The figure shows three views and two pictorial views of one solid part (mm, origin at its lowest corner). Answer the questions. A direction names the side the tool comes from. Give positions to 0.01 mm unless a question says otherwise; leave off trailing zeros. Order: outer loops, then holes, each group sorted by start corner. A loop starts at its lowest first (then second) coordinate and runs counter-clockwise, first axis right, second up. Notation, with made-up numbers: M 53,-29.75 L 105,-29.75 A16 ccw 105,-2.75 Z; hole C -39,-0.75 d9. An arc over 180 degrees is marked long. Write item = value, one per line. Start each with the question number.
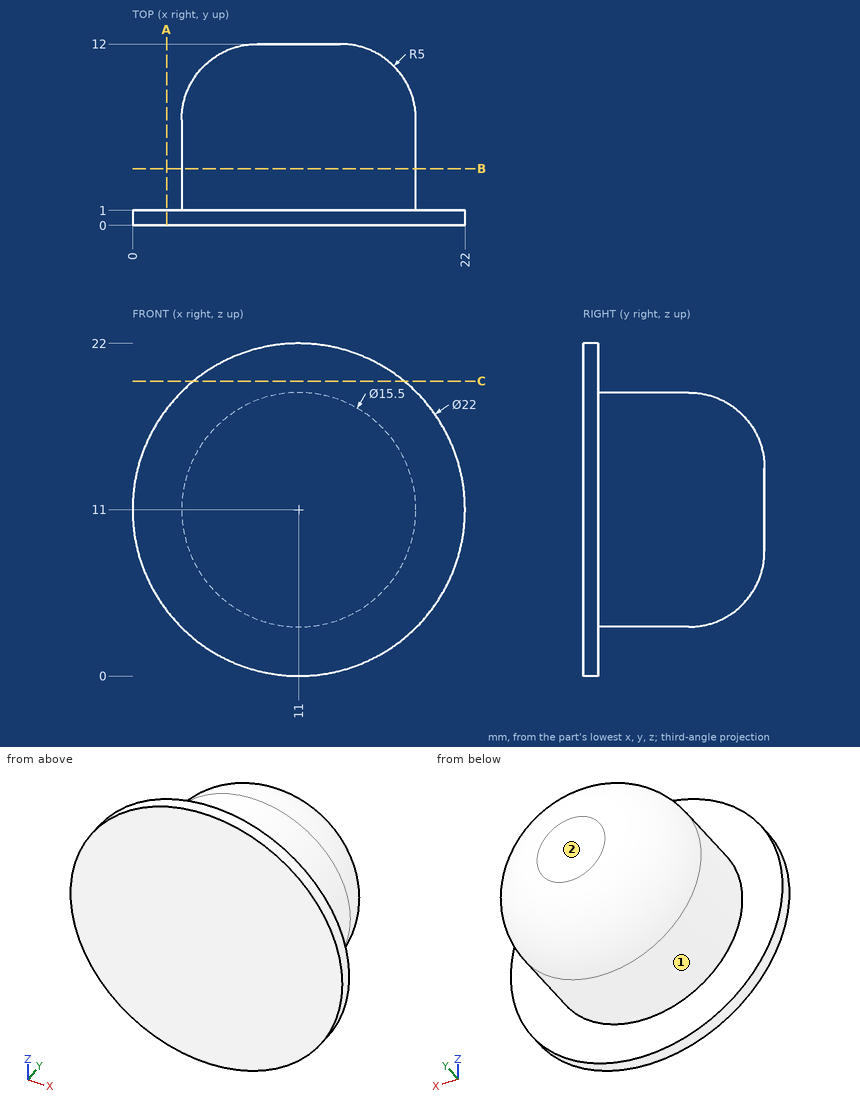
1) Find section C-C on z = 19.5. Determine the outline of the cut face in (x, y).
2) Each of these flat-tipped pins is pushed along its axis until it touches: P1, Ø3, axis at x = 11, y = 8, coming from the -Z side; P2, Ø3, axis at y = 5.5, z = 5.5, coming from the +X side; P3, Ø5, axis at x = 11.5, y = 11, coming from the +Z side. Where does it stop, or does it pass through?
3) For the marked faces 1 and 2, determine the directions among +Z, -Z, +X, -X, +Y, -Y from which every point of the face is accessible in a straight line to the end or side of a thin tool.
4) Find section B-B on y = 3.75. Determine the outline of the cut face in (x, z), plus the area to 3 significant figures.
5) Find the intervals of material crossed by probe 1 along Y at (x, z) = (4, 17.75); probe 2 along X at (y, z) = (9.75, 7.5); probe 3 along Y at (x, z) = (13.5, 4.5), in increasing order. Write a range as [from, to].
6) Find section A-A on x = 2.25. Determine the outline of the cut face in (y, z).
Numbers:
q1.outline = M 4.02,0 L 17.98,0 L 17.98,1 L 4.02,1 Z
q2.P1 = 3.25
q2.P2 = 17.64
q2.P3 = 18.51
q3.face_1 = +Y
q3.face_2 = +Z, -Z, +X, -X, +Y
q4.outline = C 11,11 d15.5
q4.area = 189 mm2
q5.probe_1 = [0, 1]
q5.probe_2 = [5.02, 16.98]
q5.probe_3 = [0, 9.69]
q6.outline = M 0,4.33 L 1,4.33 L 1,17.67 L 0,17.67 Z
